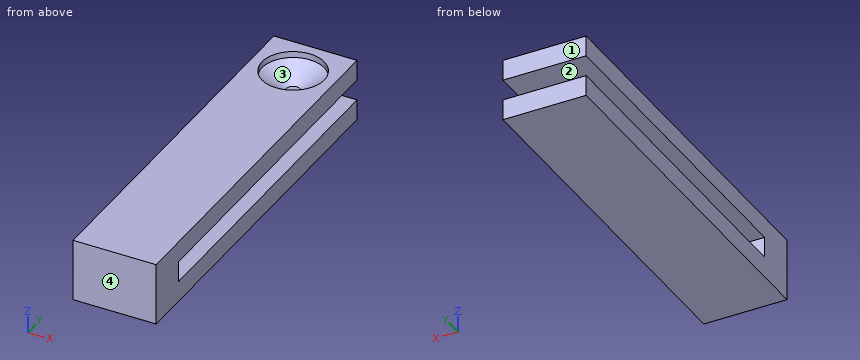
from build123d import *

# Parameters (mm, degrees)
F1_DEPTH = 50.8
F3_D     = 76.2
F3_DEPTH = 7.62
F3_TIP   = 22.892789585


with BuildPart() as f1:
    # F0 (on Right) → F1 (new body, symmetric)
    with BuildSketch(Plane.YZ):
        Polygon((285.3764565342, 50.8), (-171.8235434658, 50.8), (-171.8235434658, -25.4), (285.3764565342, -25.4), (285.3764565342, 0), (-121.0235434658, 0), (-121.0235434658, 25.4), (285.3764565342, 25.4), align=None)
    extrude(amount=F1_DEPTH, both=True)

    # F3
    with Locations(Plane.XY.offset(50.8)):
        with Locations((0, 234.5764565342)):
            Hole(F3_D / 2, depth=F3_DEPTH)
            with Locations((0, 0, -(F3_DEPTH + F3_TIP / 2))):  # 118° drill point
                Cone(0, F3_D / 2, F3_TIP, mode=Mode.SUBTRACT)


solid = f1.part
Read the model definition and answer for the solid it produces. Units are mm, in the model's axes. Face numbers are marked on the shaded views. Round coordinates to 2 decimals unless told otherwise and drop trailing zeros. Write each loop counter-clockwise with the first axis right and the second up, starting at its lowest first coordinate (ties: lowest second). Pieces come first, ordered by that corner, then holes. Notation, with made-up numbers: M 37,-17 L 77,-17 A20 cw 77,8 Z; hole C 20.5,2.5 d4. An arc over 180 degrees is marked long. Use a Markdown table: item, result.
1) The part is cut by section B-B (x = 0). Write down the section's boundary in (y, z).
Answers follow:
| item | result |
|---|---|
| outline | M -171.82,-25.4 L 285.38,-25.4 L 285.38,0 L -121.02,0 L -121.02,25.4 L 226.07,25.4 L 196.48,43.18 L 196.48,50.8 L -171.82,50.8 Z; M 243.09,25.4 L 285.38,25.4 L 285.38,50.8 L 272.68,50.8 L 272.68,43.18 Z |
2) The part is cut by section C-C (z = 35.5). Write down the section's boundary in (x, y).
Answers follow:
| item | result |
|---|---|
| outline | M -50.8,-171.82 L 50.8,-171.82 L 50.8,285.38 L -50.8,285.38 Z; hole C 0,234.58 d50.64 |
3) For a pull along Y with two mould halves and no side action, classify the marked faces 1, 2, 3 and 4 as pulls with the +Y half, pulls with the -Y half, needs draft (parallel to the pull), parting line crosses it, or undercut.
Answers follow:
| item | result |
|---|---|
| face 1 | pulls with the +Y half |
| face 2 | needs draft |
| face 3 | undercut |
| face 4 | pulls with the -Y half |
4) The part is cut by section A-A (y = 152.5). Write down the section's boundary in (x, z).
Answers follow:
| item | result |
|---|---|
| outline | M -50.8,-25.4 L 50.8,-25.4 L 50.8,0 L -50.8,0 Z; M -50.8,25.4 L 50.8,25.4 L 50.8,50.8 L -50.8,50.8 Z |
5) Straight lines are drawn through the part: line 1 along Z through (x, y) = (11.5, 13.5); line 2 along Y through (x, z) = (0, 45); line 3 along Y through (x, z) = (26.5, 2). For each, find the intervals that lie inside material, in ascending order. Write a range as [from, to].
Answers follow:
| item | result |
|---|---|
| line 1 | z = [-25.4, 0], [25.4, 50.8] |
| line 2 | y = [-171.82, 196.48], [272.68, 285.38] |
| line 3 | y = [-171.82, -121.02] |
6) The part is cut by section D-D (z = 16.5). Write down the section's boundary in (x, y).
Answers follow:
| item | result |
|---|---|
| outline | M -50.8,-171.82 L 50.8,-171.82 L 50.8,-121.02 L -50.8,-121.02 Z |
7) Flat-ended cylindrical pins translate along their axes: pin 1 (12.5 mm diameter, centred on x = 9, z = 9, fed in from +Y); pin 2 (8 mm diameter, centred on y = 44, z = 7.5, fed in from -X); pin 3 (2 mm diameter, centred on x = -23.5, y = 235, fed in from +Z). Find the tip coordinate at first contact, or state that the pin passes through.
Answers follow:
| item | result |
|---|---|
| pin 1 | stops at y = -121.02 |
| pin 2 | passes through |
| pin 3 | stops at z = 35.01 |
